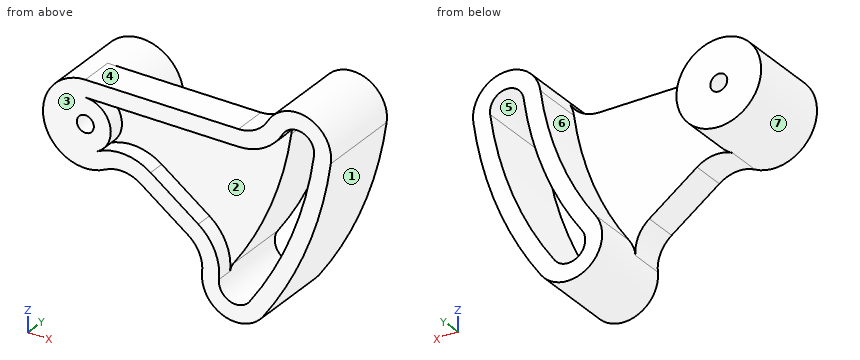
from build123d import *

# Parameters (mm, degrees)
SKETCH1_R                = 25
SKETCH1_R_2              = 5
BOSS_EXTRUDE1_DEPTH      = 50
BOSS_EXTRUDE4_DEPTH      = 20
BOSS_EXTRUDE5_DEPTH      = 30
BOSS_EXTRUDE5_DEPTH_BACK = 20
FILLET2_R                = 20
SHELL2_DEPTH             = 40
SHELL2_2_DEPTH           = 10
CUT_EXTRUDE2_DEPTH       = 171.486818667
CUT_EXTRUDE2_DEPTH_BACK  = 171.486818667


# Read off the part's stored shape, not the designer's step: Shell2
with BuildPart() as part:
    # Sketch1 → Boss-Extrude1 (new body)
    with BuildSketch(Plane(origin=(0, 0, 0), x_dir=(1, 0, 0), z_dir=(0, 1, 0))):
        with Locations(Location((0, 0, 0), (0, 0, 270))):
            Circle(SKETCH1_R)
        with Locations(Location((0, 0, 0), (0, 0, 270))):
            Circle(SKETCH1_R_2, mode=Mode.SUBTRACT)
    extrude(amount=BOSS_EXTRUDE1_DEPTH)

    # Sketch3 → Boss-Extrude4 (add)
    with BuildSketch(Plane(origin=(0, 0, 0), x_dir=(1, 0, 0), z_dir=(0, 1, 0))):
        with BuildLine():
            Line((0, -25), (125, -25))
            ThreePointArc((125, -25), (112.372583962, 21.969985307), (88.780749417, 64.502990119))
            Line((88.780749417, 64.502990119), (20.225424859, 14.694631307))
            ThreePointArc((20.225424859, 14.694631307), (23.776412907, 7.725424859), (25, 0))
            ThreePointArc((25, 0), (17.67766953, -17.67766953), (0, -25))
        make_face()
    extrude(amount=BOSS_EXTRUDE4_DEPTH)

    # Sketch4 → Boss-Extrude5 (add, two sides: drawn at the far end of the back side and taken through both)
    with BuildSketch(Plane(origin=(0, 20, 0), x_dir=(1, 0, 0), z_dir=(0, 1, 0)).offset(-BOSS_EXTRUDE5_DEPTH_BACK)):
        with BuildLine():
            ThreePointArc((144.802264946, -22.194593966), (130.912107304, 29.472389872), (104.961089304, 76.258695165))
            ThreePointArc((104.961089304, 76.258695165), (77.025044371, 80.683330007), (72.600409529, 52.747285074))
            ThreePointArc((72.600409529, 52.747285074), (93.83306062, 14.467580743), (105.197735054, -27.805406034))
            ThreePointArc((105.197735054, -27.805406034), (127.805406034, -44.802264946), (144.802264946, -22.194593966))
        make_face()
    extrude(amount=BOSS_EXTRUDE5_DEPTH + BOSS_EXTRUDE5_DEPTH_BACK)

    # Fillet2
    # the kernel refuses this fillet: 20 mm, written as the material it adds along each edge
    with BuildSketch(Plane(origin=(20.225424859, 0, -14.694631307), x_dir=(-0.7569254846609251, 0, -0.6535011940852316), z_dir=(0, 1, 0))) as fillet2_piece_1:
        with BuildLine():
            CenterArc((15.977305143, -19.472064177), FILLET2_R, 103.193899981, 63.612200039)
            Line((-3.494759034, -14.90711985), (0, 0))
            ThreePointArc((0, 0), (5.706180408, -0.659919779), (11.412360816, 0))
        make_face()
    extrude(amount=20)
    with BuildSketch(Plane(origin=(104.777715273, 20, 25), x_dir=(-1, 0, 0), z_dir=(0, -1, 0))) as fillet2_piece_2:
        with BuildLine():
            CenterArc((14.418731424, -20), FILLET2_R, 90, 60)
            Line((-2.901776652, -10), (-4.633827459, -9))
            ThreePointArc((-4.633827459, -9), (-2.400246276, -2.524865431), (-1.975559608, 0.311711782))
            Line((-1.975559608, 0.311711782), (0, 2))
            Line((0, 2), (14.418731424, 2))
            Line((14.418731424, 2), (14.418731424, 0))
        make_face()
    extrude(amount=20)
    with BuildSketch(Plane(origin=(72.600409529, 0, -52.747285074), x_dir=(-0.8090169943749511, 0, 0.5877852522924683), z_dir=(0, 1, 0))) as fillet2_piece_3:
        with BuildLine():
            CenterArc((14.641016151, -20), FILLET2_R, 90, 60)
            ThreePointArc((-2.679491924, -10), (-0.681483474, -5.176380902), (0, 0))
            Line((0, 0), (14.641016151, 0))
        make_face()
    extrude(amount=20)

    # Shell2 outline → Shell2 (cut)
    with BuildSketch(Plane(origin=(0, 0, 0), x_dir=(1, 0, 0), z_dir=(0, 1, 0))):
        with BuildLine():
            ThreePointArc((115.098867527, -26.402703017), (126.402703017, -34.901132473), (134.901132473, -23.597296983))
            ThreePointArc((134.901132473, -23.597296983), (121.642345633, 25.721187589), (96.87091936, 70.380842642))
            ThreePointArc((96.87091936, 70.380842642), (82.902896893, 72.593160063), (80.690579473, 58.625137596))
            ThreePointArc((80.690579473, 58.625137596), (103.102822291, 18.218783025), (115.098867527, -26.402703017))
        make_face()
    extrude(amount=SHELL2_DEPTH, mode=Mode.SUBTRACT)

    # Shell2 2 outline → Shell2 2 (cut)
    with BuildSketch(Plane(origin=(0, 0, 0), x_dir=(1, 0, 0), z_dir=(0, 1, 0))):
        with BuildLine():
            ThreePointArc((6.95227087, 13.291573637), (14.566633183, -3.579552727), (0, -15))
            Line((0, -15), (90.358983849, -15))
            ThreePointArc((90.358983849, -15), (105.358983849, -19.019237886), (116.339745962, -30))
            ThreePointArc((116.339745962, -30), (115.546619457, -28.260919549), (115.098867527, -26.402703017))
            ThreePointArc((115.098867527, -26.402703017), (103.102822291, 18.218783025), (80.690579473, 58.625137596))
            ThreePointArc((80.690579473, 58.625137596), (79.444945152, 60.919310624), (78.835530463, 63.457705487))
            ThreePointArc((78.835530463, 63.457705487), (76.406237331, 48.119752296), (66.633431171, 36.051341757))
            Line((66.633431171, 36.051341757), (38.49037018, 15.604211079))
            ThreePointArc((38.49037018, 15.604211079), (23.050773127, 9.955052843), (6.95227087, 13.291573637))
        make_face()
    extrude(amount=SHELL2_2_DEPTH, mode=Mode.SUBTRACT)

    # Sketch4<3> → Cut-Extrude2 (cut, two sides: drawn at the far end of the back side and taken through both)
    with BuildSketch(Plane(origin=(0, 20, 0), x_dir=(1, 0, 0), z_dir=(0, 1, 0)).offset(-CUT_EXTRUDE2_DEPTH_BACK)):
        with BuildLine():
            Line((125, -25), (114.894805022, -25))
            ThreePointArc((114.894805022, -25), (114.998144363, -25.70116121), (115.098867527, -26.402703017))
            ThreePointArc((115.098867527, -26.402703017), (126.402703017, -34.901132473), (134.901132473, -23.597296983))
            ThreePointArc((134.901132473, -23.597296983), (121.642345633, 25.721187589), (96.87091936, 70.380842642))
            ThreePointArc((96.87091936, 70.380842642), (82.902896894, 72.593160063), (80.690579473, 58.625137596))
            Line((80.690579473, 58.625137596), (88.780749417, 64.502990119))
            ThreePointArc((88.780749417, 64.502990119), (112.372583962, 21.969985307), (125, -25))
        make_face()
        with BuildLine():
            ThreePointArc((80.690579473, 58.625137596), (102.835736386, 18.875266979), (114.894805022, -25))
            Line((114.894805022, -25), (125, -25))
            ThreePointArc((125, -25), (112.372583962, 21.969985307), (88.780749417, 64.502990119))
            Line((88.780749417, 64.502990119), (80.690579473, 58.625137596))
        make_face()
    extrude(amount=CUT_EXTRUDE2_DEPTH + CUT_EXTRUDE2_DEPTH_BACK, mode=Mode.SUBTRACT)


solid = part.part
Geometry check sheet. Reference: the model listing, model coordinates, mm. Face numbers are marked on the shaded views. A direction names the side the tool comes from. Round coordinates to 2 decimals unless told otherwise and drop trailing zeros. Order: outer loops, then holes, each group sorted by start corner. A loop starts at its lowest first (then second) coordinate and runs counter-clockwise, first axis right, second up. Notation, with made-up numbers: M -6,23.25 L 40,23.25 A32 ccw 40,51.25 Z; hole C 48.25,-12 d5. An arc over 180 degrees is marked long. Answer in a Markdown table with one row per item. Add a question column.
Item 1: Sectioned sample at A-A, the plane y = 37.5. Enter the section's corners in (x, z), plus the area to 3 significant figures.
Item 2: Material ranges on L1, parallel to X at y = 18, z = -21.5; L2, parallel to X at y = 28, z = -22; L3, parallel to X at y = 24.5, z = 0, recorded low to high. Write a range as [from, to].
Item 3: Set-up check for the marked faces 4, 5, 6 and 7: record each of +Z, -Z, +X, -X, +Y, -Y from which the full face is reachable in a straight line by a thin tool's end or side.
Item 4: Sectioned sample at B-B, the plane z = -48.5. Enter the section's corners in (x, y).
Item 5: Draft check along Z on the marked faces 1, 2 and 3. Enter one of: released by +Z, released by -Z, zero draft, split by the parting line, or undercut.
Item 6: Sectioned sample at D-D, the plane z = 0. Enter the section's corners in (x, y), plus the area to 3 significant figures.
Item 7: Sectioned sample at C-C, the plane x = 132. Enter the section's corners in (y, z) (3 decimals).
Item 8: Depth check by flat-ended pin: pin 1 Ø10 at (x, y) = (61, 6.5) entering from +Z; pin 2 Ø10 at (y, z) = (27.5, -40.5) entering from -X; pin 3 Ø8 at (y, z) = (44.5, -62.5) entering from +X. Enter the tip coordinate at first touch or a pass-through.
Filled in:
| question | item | result |
|---|---|---|
| 1 | outline | C 0,0 d50; M 72.6,-52.75 A20 ccw 104.96,-76.26 A220 ccw 144.8,22.19 A20 ccw 105.2,27.81 A180 cw Z; hole C 0,0 d10; hole M 80.69,-58.63 A10 ccw 96.87,-70.38 A210 ccw 134.9,23.6 A10 ccw 115.1,26.4 A190 cw Z |
| 1 | area | 4,780 mm² |
| 2 | L1 | x = [-12.76, 12.96], [28.75, 101.74], [123.3, 133.96] |
| 2 | L2 | x = [-11.87, 11.87], [90.58, 101.53], [123.11, 133.78] |
| 2 | L3 | x = [-25, -5], [5, 25], [98.98, 109.42], [130.17, 140.48] |
| 3 | face 4 | +Z, -X, +Y, -Y |
| 3 | face 5 | +Y, -Y |
| 3 | face 6 | +Z, +Y |
| 3 | face 7 | +Y |
| 4 | outline | M 65.13,0 L 76.57,0 L 76.57,10 L 87.56,10 L 87.56,50 L 75.59,50 L 75.59,20 L 65.13,20 Z; M 110.79,0 L 122.14,0 L 122.14,50 L 110.79,50 Z |
| 5 | face 1 | released by -Z |
| 5 | face 2 | undercut |
| 5 | face 3 | zero draft |
| 6 | outline | M -25,0 L -5,0 L -5,50 L -25,50 Z; M 5,0 L 15,0 L 15,10 L 109.42,10 L 109.42,50 L 98.98,50 L 98.98,20 L 25,20 L 25,50 L 5,50 Z; M 130.17,0 L 140.48,0 L 140.48,50 L 130.17,50 Z |
| 6 | area | 3,570 mm² |
| 7 | outline | M 0,-26.731 L 50,-26.731 L 50,7.604 L 0,7.604 Z; M 0,32.141 L 50,32.141 L 50,43.735 L 0,43.735 Z |
| 8 | pin 1 | stops at z = 25 |
| 8 | pin 2 | stops at x = 77.6 |
| 8 | pin 3 | stops at x = 116.6 |
